from build123d import *

# Parameters (mm, degrees)
F0_R      = 135.89
F1_DEPTH  = 1289.304
F2_R      = 87.376
F3_DEPTH  = 120.65
F4_R      = 89.662
F5_DEPTH  = 25.4
F6_R      = 60.325
F7_DEPTH  = 1397
F9_R      = 3.937
F10_DEPTH = 762
F11_DEPTH = 762


# Not quite as in the source:
# - a fillet or chamfer that OpenCascade refuses, or shapes differently, is made with other operations: its cross-section is extruded or revolved along the edge and cut away or added


with BuildPart() as f1:
    # F0 (on Front) → F1 (new body)
    with BuildSketch(Plane.XZ):
        Circle(F0_R)
    extrude(amount=F1_DEPTH)

    # F2 (on face) → F3 (cut)
    with BuildSketch(Plane.XZ.offset(1289.304)):
        Circle(F2_R)
    extrude(amount=-F3_DEPTH, mode=Mode.SUBTRACT)

    # F4 (on face) → F5 (cut)
    with BuildSketch(Plane.XZ.offset(1289.304)):
        Circle(F4_R)
    extrude(amount=-F5_DEPTH, mode=Mode.SUBTRACT)

    # F6 (on face) → F7 (cut)
    with BuildSketch(Plane.XZ.offset(1168.654)):
        Circle(F6_R)
    extrude(amount=-F7_DEPTH, mode=Mode.SUBTRACT)

    # F8: fillet of radius 3.048 on 2 edges, made by hand

    # F8_s1 → F8_t2 (revolve)
    with BuildSketch(Plane.XY):
        with BuildLine():
            ThreePointArc((84.328, -1168.654), (86.4832614691, -1169.5467385309), (87.376, -1171.702))
            Line((87.376, -1171.702), (87.376, -1168.654))
            Line((87.376, -1168.654), (84.328, -1168.654))
        make_face()
    revolve(axis=Axis((0, -1168.654, 0), (0, -1, 0)))

    # F8_s3 → F8_t4 (revolve)
    with BuildSketch(Plane.XY):
        with BuildLine():
            ThreePointArc((89.662, -1266.8552133098), (89.023655577, -1264.9887021258), (87.376, -1263.904))
            Line((87.376, -1263.904), (89.662, -1263.904))
            Line((89.662, -1263.904), (89.662, -1266.8552133098))
        make_face()
    revolve(axis=Axis((0, -1263.904, 0), (0, -1, 0)))

    # F9 (on face) → F10 (cut)
    with BuildSketch(Plane.XZ.offset(1168.654)):
        with Locations((-60.0598781159, 39.003340895)):
            Circle(F9_R)
        with Locations((-43.0978960277, 58.6797422495)):
            Circle(F9_R)
        with Locations((-18.5348584976, 69.173033624)):
            Circle(F9_R)
        with Locations((-70.0482739288, 14.8892202572)):
            Circle(F9_R)
        with Locations((-70.7315167837, -11.2027716991)):
            Circle(F9_R)
        with Locations((-62.0188452827, -35.8065970188)):
            Circle(F9_R)
        with Locations((-53.6351113584, -47.4523380861)):
            Circle(F9_R)
        with Locations((-43.0978960277, -57.1928397463)):
            Circle(F9_R)
        with Locations((-30.8302747111, -64.6370151036)):
            Circle(F9_R)
        with Locations((-17.3247996515, -69.4859761197)):
            Circle(F9_R)
        with Locations((-3.1237236512, -71.5450341451)):
            Circle(F9_R)
        with Locations((11.2027716991, -70.7315167837)):
            Circle(F9_R)
        with Locations((37.9492110938, -60.7314328633)):
            Circle(F9_R)
        with Locations((53.218974585, -47.9185799497)):
            Circle(F9_R)
        with Locations((66.8566762325, -25.6638735077)):
            Circle(F9_R)
        with Locations((71.6131940376, 0)):
            Circle(F9_R)
        with Locations((66.8566762325, 25.6638735077)):
            Circle(F9_R)
        with Locations((32.5117097491, 63.8078231055)):
            Circle(F9_R)
    extrude(amount=-F10_DEPTH, mode=Mode.SUBTRACT)

    # F9 (on face) → F11 (cut)
    with BuildSketch(Plane.XZ.offset(1168.654)):
        with Locations((-60.0598781159, 39.003340895)):
            Circle(F9_R)
        with Locations((-43.0978960277, 58.6797422495)):
            Circle(F9_R)
        with Locations((-18.5348584976, 69.173033624)):
            Circle(F9_R)
        with Locations((-70.0482739288, 14.8892202572)):
            Circle(F9_R)
        with Locations((-70.7315167837, -11.2027716991)):
            Circle(F9_R)
        with Locations((-62.0188452827, -35.8065970188)):
            Circle(F9_R)
        with Locations((-53.6351113584, -47.4523380861)):
            Circle(F9_R)
        with Locations((-43.0978960277, -57.1928397463)):
            Circle(F9_R)
        with Locations((-30.8302747111, -64.6370151036)):
            Circle(F9_R)
        with Locations((-17.3247996515, -69.4859761197)):
            Circle(F9_R)
        with Locations((-3.1237236512, -71.5450341451)):
            Circle(F9_R)
        with Locations((11.2027716991, -70.7315167837)):
            Circle(F9_R)
        with Locations((37.9492110938, -60.7314328633)):
            Circle(F9_R)
        with Locations((53.218974585, -47.9185799497)):
            Circle(F9_R)
        with Locations((66.8566762325, -25.6638735077)):
            Circle(F9_R)
        with Locations((71.6131940376, 0)):
            Circle(F9_R)
        with Locations((66.8566762325, 25.6638735077)):
            Circle(F9_R)
        with Locations((32.5117097491, 63.8078231055)):
            Circle(F9_R)
    extrude(amount=-F11_DEPTH, mode=Mode.SUBTRACT)


solid = f1.part
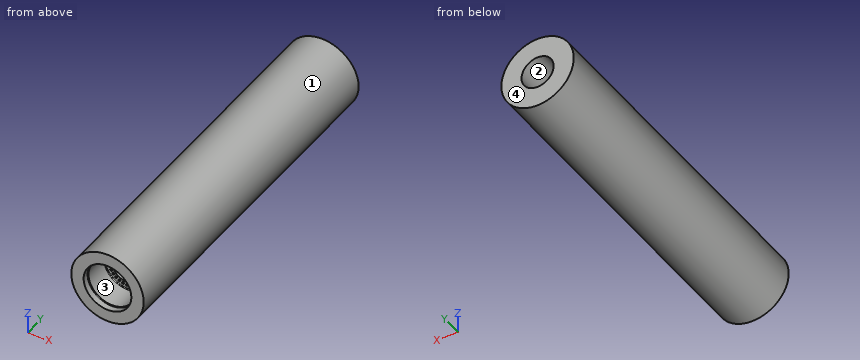
Can you work these out from the model? Positions are in its coordinate system, mm. Face numbers are marked on the shaded views. Give positions to 0.01 mm unless a question says otherwise; leave off trailing zeros. Loops run counter-clockwise (first coordinate to the right, second up) from the corner with the lowest first, then second, coordinate; pieces in that order, holes last. Notation, with made-up numbers: (-2.5, -13.75) - (32.5, -13.75) arc R22 cw to (32.5, 13.25) - close; hole circle Ø3 at (65.25, 35). An arc over 180 degrees is marked (long way). Answer as a JSON object with one key per item and string values.
Q1. Imagine slicing it at B-B on y = -1138.5. Give the number of separate pieces and of enclosed holes in the cut face, plus the area to 3 significant figures.
Geometry says:
{"separate pieces": "1", "enclosed holes": "19", "area": "45,700 mm²"}
Q2. Will these pins go through, and if not, where does the flat tip stop? P1, Ø10, axis at x = 66.86, z = -25.66, coming from the -Y side; P2, Ø4.5, axis at x = 32.51, z = 63.81, coming from the -Y side; P3, Ø4, axis at y = -263.5, z = -62, coming from the +X side.
Geometry says:
{"P1": "y = -1168.65", "P2": "y = -406.65", "P3": "x = 121.93"}
Q3. If I drill on L1, parallel to X at y = -819, z = -1; L2, parallel to Z at x = 68.5, y = -1096; L3, parallel to X at y = -1064, z = -74, over which ranges is the centre line in solid material (lowest first)?
Geometry says:
{"L1": "-135.89 to -60.32, 60.32 to 67.81, 75.42 to 135.89", "L2": "-117.36 to -29.24, -22.09 to -2.41, 2.41 to 22.09, 29.24 to 117.36", "L3": "-113.97 to -6.2, -0.05 to 9.01, 13.4 to 113.97"}
Q4. Imagine slicing it at A-A on y = -262. Write out the boundary of the cut face in (x, z) (3 decimals), plus the area to 3 significant figures.
Geometry says:
{"outline": "circle Ø271.78 at (0, 0); hole circle Ø120.65 at (0, 0)", "area": "46,600 mm²"}
Q5. If we mould it in two halves opening along X, with no side actions, what happens to the marked faces 1, 2, 3 and 4? For each: pulls with the +X half, pulls with the -X half, needs draft (parallel to the pull), parting line crosses it, or undercut.
Geometry says:
{"face 1": "parting line crosses it", "face 2": "undercut", "face 3": "undercut", "face 4": "needs draft"}
Q6. Imagine slicing it at C-C on x = -119. Write out the boundary of the cut face in (y, z), plus the area to 3 significant figures.
Geometry says:
{"outline": "(-1289.3, -65.61) - (0, -65.61) - (0, 65.61) - (-1289.3, 65.61) - close", "area": "169,000 mm²"}
